Autodesk Inventor part; units mm, degrees
ref_plane "XZ Plane" through (0, 0, 0) normal (0, 1, 0) x (-1, 0, 0)
ref_plane "XY Plane" through (0, 0, 0) normal (0, 0, 1) x (1, 0, 0)
sketch "Sketch1" plane through (0, 0, 0) normal (0, 0, 1) x (1, 0, 0)
  circle A0 centre (0, 0) radius 40
  dimension "d0" = 80
extrude "Extrusion1" add sketch "Sketch1" along normal blind 4
ref_plane "Work Plane2" through (10, 0, 0) normal (1, 0, 0) x (0, 1, 0)
ref_plane "Work Plane1" through (-40, 0, 0) normal (1, 0, 0) x (0, 1, 0)
sketch "Sketch2" plane through (10, 0, 0) normal (1, 0, 0) x (0, 1, 0)
  line L0 (-21.6965, 0) -> (-21.6965, -5)
  line L1 (-21.6965, -5) -> (28.3035, -5)
  line L2 (28.3035, -5) -> (28.3035, 0)
  circle A0 centre (13.3035, -44.0044) radius 10
  line L3 (-21.6965, -5) -> (0, -41.2491)
  line L4 (28.3035, -5) -> (23.2249, -45.256)
  line L5 (-21.6965, 0) -> (28.3035, 0)
  line L6 (28.3035, -5) -> (28.3035, -63.6411)
  arc A1 (0, -69.0405) -> (28.3035, -60.1475) centre (13.3035, -61.8943) ccw
  arc A2 (4.8652, -49.3705) -> (4.8622, -49.3725) centre (13.3035, -61.8943) ccw
  line L7 (0, -69.0405) -> (-21.6965, -5)
  point P0 (0, 0)
  point P1 (11.1199, -34.2457)
  point P2 (4.723, -49.1401)
  dimension "d4" = 5
  dimension "d5" = 50
  dimension "d6" = 20
  dimension "d8" = 15
extrude "Extrusion4" add sketch "Sketch2" along normal blind 5 contours L5 L2 L1 L0 | L1 L6 A1 L7 | A0
sketch "Sketch3" plane through (10, 0, 0) normal (-1, 0, 0) x (0, 0, 1)
  arc A0 (-45.256, 23.2249) -> (-49.1401, 4.723) centre (-44.0044, 13.3035) ccw
  circle A1 centre (-44.0044, 13.3035) radius 6.4
  point P0 (0, 0)
  dimension "d15" = 12.8
extrude "Extrusion5" cut sketch "Sketch3" against normal through all
sketch "Sketch6" plane through (15, 0, 0) normal (1, 0, 0) x (0, 0, -1)
  point P0 (0, 0)
sketch "Sketch7" plane through (15, 0, 0) normal (1, 0, 0) x (0, 0, -1)
  line L0 (13.4044, 3.4035) -> (54.0044, 3.4035)
  line L1 (54.0044, 3.4035) -> (54.0044, 23.2035)
  line L2 (54.0044, 23.2035) -> (13.4044, 23.2035)
  line L3 (13.4044, 23.2035) -> (13.4044, 3.4035)
  line L4 (13.4044, 3.4035) -> (54.0044, 23.2035) construction
  line L5 (54.0044, 3.4035) -> (13.4044, 23.2035) construction
  circle A0 centre (44.0044, 13.3035) radius 6.4
  point P0 (0, 0)
  point P1 (33.7044, 13.3035)
  dimension "d24" = 40.6
  dimension "d25" = 19.8
  dimension "d35" = 9.9
  dimension "d36" = 10
extrude "Extrusion8" cut sketch "Sketch7" against normal blind 2 contours L3 L2 L1 L0 | A0
sketch "Sketch8" plane through (15, 0, 0) normal (1, 0, 0) x (0, 0, -1)
  line L0 (54.0044, 23.2035) -> (54.0044, 3.4035)
  line L1 (54.0044, 23.2035) -> (64.0044, 23.2035)
  line L2 (64.0044, 23.2035) -> (64.0044, 3.4035)
  line L3 (64.0044, 3.4035) -> (54.0044, 3.4035)
  line L4 (54.0044, 3.4035) -> (54.0044, 23.2035)
  point P0 (0, 0)
  dimension "d28" = 10
  dimension "d29" = 19.8
extrude "Extrusion9" add sketch "Sketch8" along normal blind 5.5
sketch "Sketch9" plane through (15, 0, 0) normal (1, 0, 0) x (0, 0, -1)
  line L0 (64.0044, 23.2035) -> (64.0044, 3.4035)
  line L1 (64.0044, 23.2035) -> (70.7533, 23.2035)
  line L2 (70.7533, 23.2035) -> (70.7533, 3.4035)
  line L3 (70.7533, 3.4035) -> (64.0044, 3.4035)
  line L4 (64.0044, 3.4035) -> (64.0044, 23.2035)
  point P0 (0, 0)
extrude "Extrusion10" add sketch "Sketch9" along normal blind 5.5
fillet "Fillet1" radius 10 1 edges at (20.5, 13.3035, -70.7533)
sketch "Sketch10" plane through (15, 0, 0) normal (1, 0, 0) x (0, 0, -1)
  line L0 (13.4044, 3.4035) -> (13.4044, 23.2035)
  line L1 (13.4044, 3.4035) -> (13.4044, 23.2035)
  line L2 (13.4044, 23.2035) -> (0.0004, 23.2035)
  line L3 (0.0004, 23.2035) -> (0.0004, 3.4035)
  line L4 (0.0004, 3.4035) -> (13.4044, 3.4035)
  line L5 (13.4044, 3.4035) -> (13.4044, 23.2035)
  point P0 (0, 0)
  dimension "d38" = 13.404
extrude "Extrusion11" add sketch "Sketch10" along normal blind 5.5
sketch "Sketch11" plane through (20.5, 0, 0) normal (1, 0, 0) x (0, 0, -1)
  line L0 (0.0004, 23.2035) -> (13.4044, 23.2035)
  line L1 (13.4044, 23.2035) -> (8.8144, 23.2035)
  line L2 (13.4044, 18.3035) -> (13.4044, 23.2035)
  circle A0 centre (8.8144, 18.3035) radius 1.475
  line L3 (13.4044, 3.4035) -> (13.4044, 23.2035)
  line L4 (13.4044, 13.3035) -> (0.0004, 13.3035)
  line L5 (0.0004, 3.4035) -> (0.0004, 23.2035)
  circle A1 centre (8.8144, 8.3035) radius 1.475
  point P0 (0, 0)
  dimension "d43" = 2.95
  dimension "d44" = 2.95
extrude "Extrusion12" cut sketch "Sketch11" against normal blind 10 contours A0 | A1
sketch "Sketch12" plane through (20.5, 0, 0) normal (1, 0, 0) x (0, 0, -1)
  point P0 (0, 0)
sketch "Sketch13" plane through (10.5, 18.3035, -8.8144) normal (1, 0, 0) x (0, 0, -1)
  point P0 (-8.8144, -18.3035)
sketch "Sketch14" plane through (13, 0, 0) normal (1, 0, 0) x (0, 0, -1)
  circle A0 centre (8.8144, 18.3035) radius 1.475
  line L0 (61.7531, 18.3035) -> (54.0044, 18.3035)
  line L1 (54.0044, 23.2035) -> (54.0044, 3.4035)
  point P0 (0, 0)
sketch "Sketch15" plane through (20.5, 0, 0) normal (1, 0, 0) x (0, 0, -1)
  circle A0 centre (8.8144, 18.3035) radius 1.475
  line L0 (61.823, 23.2035) -> (61.823, 3.4035)
  circle A1 centre (8.8144, 8.3035) radius 1.475
  line L1 (54.0044, 23.2035) -> (54.0044, 3.4035)
  circle A2 centre (58.5944, 18.3035) radius 1.475
  circle A3 centre (58.5944, 8.3035) radius 1.475
  point P0 (0, 0)
  dimension "d49" = 2.95
  dimension "d50" = 2.95
extrude "Extrusion13" cut sketch "Sketch15" against normal blind 10 contours A2 | A3
thread "Thread1"
thread "Thread2"
thread "Thread3"
thread "Thread4"
sketch "Sketch16" plane through (13, 0, 0) normal (1, 0, 0) x (0, 0, -1)
  point P0 (0, 0)
sketch "Sketch17" plane through (13, 0, 0) normal (1, 0, 0) x (0, 0, -1)
  point P0 (0, 0)
sketch "Sketch18" plane through (20.5, 0, 0) normal (1, 0, 0) x (0, 0, -1)
  point P0 (0, 0)
sketch "Sketch19" plane through (13, 0, 0) normal (1, 0, 0) x (0, 0, -1)
  point P0 (0, 0)
sketch "Sketch20" plane through (13, 0, 0) normal (1, 0, 0) x (0, 0, -1)
  point P0 (0, 0)
sketch "Sketch21" plane through (0, 0, 0) normal (0, 0, -1) x (-1, 0, 0)
  circle A0 centre (0, 0) radius 6.4
  dimension "d61" = 12.8
extrude "Extrusion14" cut sketch "Sketch21" against normal blind 10
sketch "Sketch22" plane through (13, 0, 0) normal (1, 0, 0) x (0, 0, -1)
  point P0 (0, 0)
sketch "Sketch23" plane through (0, 0, 0) normal (0, 0, -1) x (-1, 0, 0)
  point P0 (0, 0)
sketch "Sketch24" plane through (0, 0, 0) normal (0, 0, -1) x (-1, 0, 0)
  point P0 (0, 0)
sketch "Sketch25" plane through (0, 0, 0) normal (0, 0, -1) x (-1, 0, 0)
  point P0 (0, 0)
properties part number "wrist" material "Aluminum 6061"
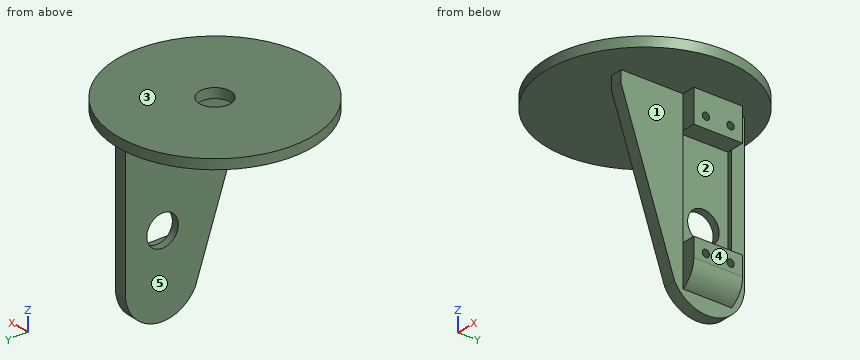
CAD build for the part. Positions are in the model's coordinates, mm. Face numbers are marked on the shaded views. A direction names the side the tool comes from. Coordinates: 2 decimals unless noted, no trailing zeros. Order: outer loops, then holes, each group sorted by start corner. A loop starts at its lowest first (then second) coordinate and runs counter-clockwise, first axis right, second up. Notation, with made-up numbers: M 39.25,36.5 L 59.25,36.5 A8 cw 59.25,43.5 Z; hole C 1,83.5 d2. An arc over 180 degrees is marked long. Write each question's results on one line, items separated by ' | '. Start each with the question number.
Q1. Pull direction Y, two halves, no side cores. Call the marked faces 1 and 2: +Y half, -Y half, draft (parallel to the pull), parting line (faces both ways), or undercut.
Q2. Drill centre lines: probe 1 along Z at (x, y) = (11.5, -37); probe 2 along X at (y, z) = (15.5, -16.5); probe 3 along X at (y, z) = (25, -16.5). Where is each one in solid material? Low to high. Write a range as from..to.
Q3. Cut at A-A (x = 0). List the corners of the cut face in (y, z).
Q4. Cut at B-B (x = 16.5). Count the separate pieces of the cut face and the enclosed holes in it, then the cut area to 3 significant figures.
Q5. Cut at D-D (x = -14.5). List the corners of the cut face in (y, z).
Q6. Cut at C-C (z = -15). List the corners of the cut face in (x, y).
Q7. Flat gauge pins, fed straight in: P1, Ø2, axis at x = 17.5, y = 17.5, coming from the -Z side; P2, Ø4, axis at y = 18.3, z = -58.59, coming from the -X side; P3, Ø8, axis at y = -3, z = -20, coming from the +X side. Where does each tip first touch, or does it go through?
Q8. Which spindle directions (+Z, -Z, +X, -X, +Y, -Y) get a long thin tool onto all of the face, cutting with end or side? Do the marked faces 3, 4 and 5. Say none if no direction does.
Found:
1) face 1: draft | face 2: undercut
2) probe 1: 0..4 | probe 2: 10..13 | probe 3: 10..15
3) outline: M -40,0 L -6.4,0 L -6.4,4 L -40,4 Z; M 6.4,0 L 40,0 L 40,4 L 6.4,4 Z
4) separate pieces: 3 | enclosed holes: 4 | area: 843 mm²
5) outline: M -37.28,0 L 37.28,0 L 37.28,4 L -37.28,4 Z
6) outline: M 10,-18.31 L 15,-18.31 L 15,3.4 L 13,3.4 L 13,23.2 L 15,23.2 L 15,28.3 L 10,28.3 Z
7) P1: z = -69.82 | P2: x = 10 | P3: x = 15
8) face 3: +Z, +X, -X, +Y, -Y | face 4: -Z, +X, +Y, -Y | face 5: -Z, -X, +Y, -Y
